Check sheet for the modelled part. Datum: model origin and axes. Units: mm. Face numbers are marked on the shaded views. A direction names the side the tool comes from. Coordinates: 2 decimals unless noted, no trailing zeros. Loops run counter-clockwise (first coordinate to the right, second up) from the corner with the lowest first, then second, coordinate; pieces in that order, holes last. Notation, with made-up numbers: (-37.5, 84.5) -> (-28.5, 84.5) arc R34 ccw to (-28.5, 116.5) -> close; hole circle Ø10 at (-10.5, 15). An arc over 180 degrees is marked (long way). Use one line per item in the form item = value.
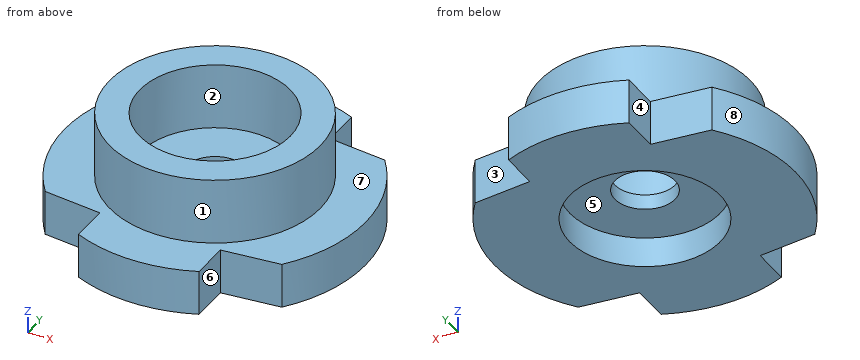
from build123d import *

# Parameters (mm, degrees)
BOSS_EXTRUDE1_DEPTH = 1.5
SKETCH2_R           = 3.5
SKETCH2_R_2         = 2.5
BOSS_EXTRUDE2_DEPTH = 2.2
CUT_EXTRUDE1_REACH  = 20.87
SKETCH3_R           = 1
SKETCH4_R           = 2.5
CUT_EXTRUDE2_DEPTH  = 1
CUT_EXTRUDE4_START  = -1.5
SKETCH5_R           = 17.5
SKETCH5_R_2         = 5
CUT_EXTRUDE4_DEPTH  = 1.5


with BuildPart() as part:
    # Sketch1 → Boss-Extrude1 (new body)
    with BuildSketch(Plane.XY):
        with BuildLine():
            Line((2, 7.75863865), (2, 3.304737557))
            Line((2, 3.304737557), (14.214285714, 1.988487272))
            ThreePointArc((14.214285714, 1.988487272), (16, 0), (14.214285714, -1.988487272))
            Line((14.214285714, -1.988487272), (2, -3.304737557))
            Line((2, -3.304737557), (2, -7.75863865))
            ThreePointArc((2, -7.75863865), (0, -9.75863865), (-2, -7.75863865))
            Line((-2, -7.75863865), (-2, -3.304737557))
            Line((-2, -3.304737557), (-14.214285714, -1.988487272))
            ThreePointArc((-14.214285714, -1.988487272), (-16, 0), (-14.214285714, 1.988487272))
            Line((-14.214285714, 1.988487272), (-2, 3.304737557))
            Line((-2, 3.304737557), (-2, 7.75863865))
            ThreePointArc((-2, 7.75863865), (0, 9.75863865), (2, 7.75863865))
        make_face()
    extrude(amount=BOSS_EXTRUDE1_DEPTH)

    # Sketch2 → Boss-Extrude2 (add)
    with BuildSketch(Plane.XY.offset(1.5)):
        Circle(SKETCH2_R)
        Circle(SKETCH2_R_2, mode=Mode.SUBTRACT)
    extrude(amount=BOSS_EXTRUDE2_DEPTH)

    # Sketch3 → Cut-Extrude1 (cut, up to next)
    with BuildSketch(Plane.XY.offset(1.5), mode=Mode.PRIVATE) as cut_extrude1_sk1:
        Circle(SKETCH3_R)
    cut_extrude1_tool1 = extrude(cut_extrude1_sk1.sketch, amount=-CUT_EXTRUDE1_REACH, mode=Mode.PRIVATE) & part.part
    add(cut_extrude1_tool1.solids().sort_by_distance((0, 0, 1.5))[0], mode=Mode.SUBTRACT)

    # Sketch4 → Cut-Extrude2 (cut)
    with BuildSketch(Plane(origin=(0, 0, 0), x_dir=(-1, 0, 0), z_dir=(0, 0, -1))):
        with Locations(Location((0, 0, 0), (0, 0, 180))):
            Circle(SKETCH4_R)
    extrude(amount=-CUT_EXTRUDE2_DEPTH, mode=Mode.SUBTRACT)

    # Sketch5 → Cut-Extrude4 (cut)
    with BuildSketch(Plane.XY.offset(1.5).offset(CUT_EXTRUDE4_START)):
        Circle(SKETCH5_R)
        Circle(SKETCH5_R_2, mode=Mode.SUBTRACT)
    extrude(amount=CUT_EXTRUDE4_DEPTH, mode=Mode.SUBTRACT)


solid = part.part
(1) Scan lines: line 1 along Z through (x, y) = (0.5, -1.5); line 2 along Y through (x, z) = (-0.75, 3.35); line 3 along X through (y, z) = (-2.25, 0.45). Record each from-to range of solid material in increasing order.
Established:
line_1 = 1 to 1.5
line_2 = -3.42 to -2.38, 2.38 to 3.42
line_3 = -4.47 to -1.09, 1.09 to 4.47
(2) Section check A-A, the plane x = 0. Record the boundary of the cut face in (y, z).
Established:
outline = (-5, 0) -> (-2.5, 0) -> (-2.5, 1) -> (-1, 1) -> (-1, 1.5) -> (-2.5, 1.5) -> (-2.5, 3.7) -> (-3.5, 3.7) -> (-3.5, 1.5) -> (-5, 1.5) -> close; (1, 1) -> (2.5, 1) -> (2.5, 0) -> (5, 0) -> (5, 1.5) -> (3.5, 1.5) -> (3.5, 3.7) -> (2.5, 3.7) -> (2.5, 1.5) -> (1, 1.5) -> close
(3) Mould release check, pull along Y, two halves, no side actions. Record for the marked faces 1, 2 and 3: +Y half, -Y half, draft (parallel to the pull), parting line (faces both ways), or undercut.
Established:
face_1 = parting line
face_2 = undercut
face_3 = +Y half
(4) Section check D-D, the plane x = -4.5. Record the boundary of the cut face in (y, z).
Established:
outline = (-2.18, 0) -> (2.18, 0) -> (2.18, 1.5) -> (-2.18, 1.5) -> close
(5) Section check C-C, the plane z = 1.95. Record the boundary of the cut face in (x, y).
Established:
outline = circle Ø7 at (0, 0); hole circle Ø5 at (0, 0)
(6) Tool access check on the marked faces 4, 5, 6, 7 and 8. Record the directions out of +Z, -Z, +X, -X, +Y, -Y that give a thin tool (end or side, any length) a straight path to the whole face; none if there is none.
Established:
face_4 = +Z, -Z, -X, +Y
face_5 = -Z
face_6 = +Z, -Z, +X, -Y
face_7 = +Z
face_8 = +Z, -Z, -X
(7) Go/stop test with flat-tipped pins: P1, Ø2.5, axis at x = 0, y = 0, coming from the -Z side; P2, Ø1, axis at y = 4, z = 1, coming from the +X side; P3, Ø1, axis at x = 1.5, y = 0, coming from the +Z side. Record where each tip stops, or that it passes through.
Established:
P1 = 1
P2 = 2
P3 = 1.5
